Autodesk Inventor part; units mm, degrees
ref_plane "YZ Plane" through (0, 0, 0) normal (1, 0, 0) x (0, 1, 0)
ref_plane "XZ Plane" through (0, 0, 0) normal (0, 1, 0) x (-1, 0, 0)
ref_plane "XY Plane" through (0, 0, 0) normal (0, 0, 1) x (1, 0, 0)
sketch "Sketch1" plane through (0, 0, 0) normal (0, 0, 1) x (1, 0, 0)
  line L0 (-175, 150) -> (175, 150)
  line L1 (175, 150) -> (175, -150)
  line L2 (175, -150) -> (-175, -150)
  line L3 (-175, -150) -> (-175, 150)
  line L4 (-175, 150) -> (175, -150) construction
  point P0 (0, 0)
  point P1 (0, 0)
  dimension "d0" = 350
  dimension "d1" = 300
extrude "Plate1" add sketch "Sketch1" against normal blind 3
sketch "Sketch2" plane through (0, 0, 0) normal (0, 0, 1) x (1, 0, 0)
  line L0 (175, -150) -> (175, 150)
  line L1 (-135, 103) -> (-135, -103) construction
  line L2 (-175, 150) -> (-175, -150)
  point P0 (0, 0)
  point P1 (-135, 0)
  dimension "d23" = 40
  dimension "d24" = 206
hole "Hole4" at (-135, 103, 0) at (-135, -103, 0) direction (0, 0, -1) diameter 12 end through all
sketch "Sketch3" plane through (0, 0, 0) normal (0, 0, 1) x (1, 0, 0)
  line L0 (-160, 135) -> (160, 135) construction
  line L1 (160, 135) -> (160, -135) construction
  line L2 (160, -135) -> (-160, -135) construction
  line L3 (-160, -135) -> (-160, 135) construction
  line L4 (-160, 135) -> (160, -135) construction
  point P0 (0, 0)
  point P1 (0, 0)
  dimension "d14" = 270
  dimension "d15" = 320
hole "Hole2" at (-160, 135, 0) at (160, 135, 0) at (160, -135, 0) at (-160, -135, 0) direction (0, 0, -1) diameter 10 end through all
sketch "Sketch4" plane through (-175, -147, 0) normal (0, -1, 0) x (1, 0, 0)
  line L0 (350, 0) -> (0, 0)
  line L1 (0, 0) -> (0, -25)
  line L2 (0, -25) -> (350, -25)
  line L3 (350, -25) -> (350, 0)
edge flange "Flange1" height 25 angle 90 thickness 3 bend radius 5 thickness toward (0, -1, 0) relief round relief width 3 relief depth 1.5 corner gap 5 corner form 0 edges at (0, -150, -3) (0, 150, -3) wall of the first edge with corners at (175, -147, 0) (-175, -147, 0) (-175, -147, -25) (175, -147, -25)
bend "Bend1"
corner "Corner1"
equation "\"d2\" = Thickness"
equation "\"d39\" = BendReliefWidth"
equation "\"d40\" = BendReliefDepth"
equation "\"d41\" = MinimumRemnant"
equation "\"d42\" = TransitionRadius"
equation "\"d45\" = BendRadius"
equation "\"d46\" = CornerReliefSize"
equation "\"d47\" = GapSize"
equation "\"d48\" = JacobiRadiusSize"
equation "\"BendReliefWidth\" = Thickness"
equation "\"BendReliefDepth\" = 0.5 * Thickness"
equation "\"CornerReliefSize\" = 4 * Thickness"
equation "\"MinimumRemnant\" = 2 * Thickness"
equation "\"TransitionRadius\" = BendRadius"
equation "\"JacobiRadiusSize\" = BendRadius"
equation "\"GapSize\" = Thickness"
properties part number "CP-190 plate" material "Stainless Steel"
For this review, take the finished solid that the model builds, in its own axes (mm). A direction names the side the tool comes from. Round coordinates to 2 decimals unless told otherwise and drop trailing zeros. Write each loop counter-clockwise with the first axis right and the second up, starting at its lowest first coordinate (ties: lowest second). Pieces come first, ordered by that corner, then holes. Notation, with made-up numbers: (13, 77) - (27, 77) arc R33 ccw to (27, 110) - close; hole circle Ø4 at (-1, 70.25). An arc over 180 degrees is marked (long way). Write item = value, one per line. Start each with the question number.
1. Consider section A-A on y = -135. State the section outline as (x, z) points.
2. For pin 1 Ø3 at (x, y) = (-108.5, 47.5) entering from -Z; pin 2 Ø1 at (x, z) = (85.5, -4) entering from -Y, all flat-tipped, find the tip position at first contact; note any pin that passes through.
3. Consider section B-B on x = -135. State the section outline as (y, z) points, plus the area to 3 significant figures.
4. Consider section D-D on y = 103. State the section outline as (x, z) points, plus the area to 3 significant figures.
5. Draft analysis for pull direction Y (two halves, no side actions). For faces 3 (the face through (-2.45, -147.719, -2.406)), 4 (the face through (2.45, 147.719, -2.406)), 5 (the face through (-2, -147, -16)), state which applies: released by +Y, released by -Y, zero draft, split by the parting line, or undercut.
6. Wall thickness on L1, parallel to Y at x = -160, z = -1.7; L2, parallel to X at y = 135, z = -1; L3, parallel to X at y = 103, z = -0.75: over which ranges is each line inside the solid? List them lowest first.
7. Consider section C-C on z = -19.25. State the section outline as (x, y) points, plus the area to 3 significant figures.
8. For faces 1 (the face through (-155.564, 132.693, -1.521)), 2 (the face through (-2, 2, -3)), list the 3-axis set-ups (+Z, -Z, +X, -X, +Y, -Y) from which the entire face can be reached by the end or side of a thin tool; tool diameter is ignored.
Evaluation:
q1.outline = (-175, -3) - (-165, -3) - (-165, 0) - (-175, 0) - close; (-155, -3) - (155, -3) - (155, 0) - (-155, 0) - close; (165, -3) - (175, -3) - (175, 0) - (165, 0) - close
q2.pin_1 = -3
q2.pin_2 = -149.19
q3.outline = (-150, -25) - (-147, -25) - (-147, -8) arc R5 cw to (-142, -3) - (-109, -3) - (-109, 0) - (-142, 0) arc R8 ccw to (-150, -8) - close; (-97, -3) - (97, -3) - (97, 0) - (-97, 0) - close; (109, -3) - (142, -3) arc R5 cw to (147, -8) - (147, -25) - (150, -25) - (150, -8) arc R8 ccw to (142, 0) - (109, 0) - close
q3.area = 943 mm2
q4.outline = (-175, -3) - (-141, -3) - (-141, 0) - (-175, 0) - close; (-129, -3) - (175, -3) - (175, 0) - (-129, 0) - close
q4.area = 1,010 mm2
q5.face_3 = released by -Y
q5.face_4 = released by +Y
q5.face_5 = undercut
q6.L1 = -146.93 to -140, -130 to 130, 140 to 146.93
q6.L2 = -175 to -165, -155 to 155, 165 to 175
q6.L3 = -175 to -141, -129 to 175
q7.outline = (-175, -150) - (175, -150) - (175, -147) - (-175, -147) - close; (-175, 147) - (175, 147) - (175, 150) - (-175, 150) - close
q7.area = 2,100 mm2
q8.face_1 = +Z, -Z
q8.face_2 = -Z, +X, -X
